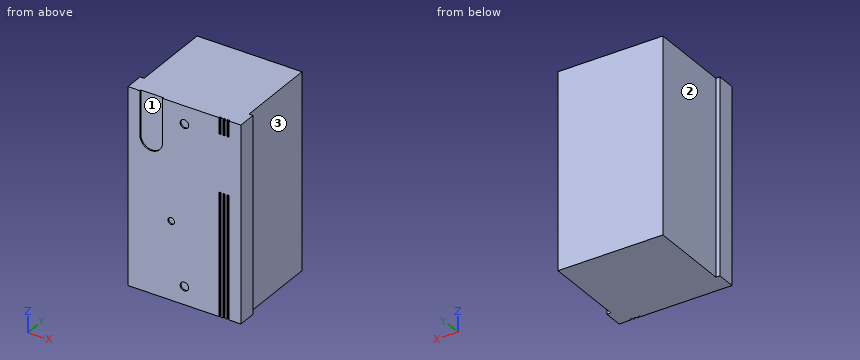
from build123d import *

# Parameters (mm, degrees)
F0_W     = 85
F0_H     = 147
F1_DEPTH = 75
F2_W     = 1.5
F2_H     = 92
F2_R     = 3.213136
F2_R_2   = 2.5
F2_H_2   = 12
F3_DEPTH = 1
F4_W     = 61
F4_H     = 147
F5_DEPTH = 3
F6_W     = 61
F6_H     = 147
F7_DEPTH = 3


with BuildPart() as f1:
    # F0 (on Front) → F1 (new body)
    with BuildSketch(Plane.XZ):
        Rectangle(F0_W, F0_H)
    extrude(amount=F1_DEPTH)

    # F2 (on face) → F3 (cut)
    with BuildSketch(Plane.XZ.offset(75)):
        with Locations((26.781611, -27.5)):
            Rectangle(F2_W, F2_H)
        with Locations((29.781611, -27.5)):
            Rectangle(F2_W, F2_H)
        with Locations((32.781611, -27.5)):
            Rectangle(F2_W, F2_H)
        with Locations((0, -60)):
            Circle(F2_R)
        with Locations((-10, -15)):
            Circle(F2_R_2)
        with Locations((0, 60)):
            Circle(F2_R)
        with BuildLine():
            Line((-16.484489, 73.5), (-33.484489, 73.5))
            Line((-33.484489, 73.5), (-33.484489, 40.5))
            ThreePointArc((-33.484489, 40.5), (-24.984489, 32), (-16.484489, 40.5))
            Line((-16.484489, 40.5), (-16.484489, 73.5))
        make_face()
        with Locations((26.781611, 67.5)):
            Rectangle(F2_W, F2_H_2)
        with Locations((29.781611, 67.5)):
            Rectangle(F2_W, F2_H_2)
        with Locations((32.781611, 67.5)):
            Rectangle(F2_W, F2_H_2)
    extrude(amount=-F3_DEPTH, mode=Mode.SUBTRACT)

    # F4 (on face) → F5 (cut)
    with BuildSketch(Plane(origin=(-42.5, 0, 0), x_dir=(0, -1, 0), z_dir=(-1, 0, 0))):
        with Locations((30.5, 0)):
            Rectangle(F4_W, F4_H)
    extrude(amount=-F5_DEPTH, mode=Mode.SUBTRACT)

    # F6 (on face) → F7 (cut)
    with BuildSketch(Plane.YZ.offset(42.5)):
        with Locations((-30.5, 0)):
            Rectangle(F6_W, F6_H)
    extrude(amount=-F7_DEPTH, mode=Mode.SUBTRACT)


solid = f1.part
Can you work these out from the model? Positions are in its coordinate system, mm. Face numbers are marked on the shaded views. A direction names the side the tool comes from. Give positions to 0.01 mm unless a question says otherwise; leave off trailing zeros. Write each loop counter-clockwise with the first axis right and the second up, starting at its lowest first coordinate (ties: lowest second). Pieces come first, ordered by that corner, then holes. Notation, with made-up numbers: (-35, 20.25) -> (-29, 20.25) arc R24 cw to (-29, 36.25) -> close; hole circle Ø2 at (56.5, 12.25). An arc over 180 degrees is marked (long way). Answer as a JSON object with one key per item and string values. Group by question number.
Item 1: I'm going to push flat-ended pins straight in: P1, Ø2, axis at y = -45.5, z = -56, coming from the +X side; P2, Ø5, axis at x = 0, z = 60, coming from the -Y side; P3, Ø0.8, axis at x = 33, y = -74.5, coming from the -Z side; P4, Ø1.6, axis at x = 33, z = 68.5, coming from the -Y side. Where does each tip first touch, or does it pass through?
Item 2: Please list where these lines run through material, in increasing order: line 1 (Z direction, x = 0, y = -74.25); line 2 (X direction, y = -37.5, z = 37); line 3 (Z direction, x = -10, y = -74.35). Write a range as [from, to].
Item 3: Suppose I cut it at D-D (z = -15). Please give me the cut outline in (x, y), plus the area to 3 significant figures.
Item 4: Suppose I cut it at A-A (z = 49.5). Please give me the cut outline in (x, y), plus the area to 3 significant figures.
Item 5: Suppose I cut it at C-C (z = -60). Please give me the cut outline in (x, y).
Item 6: For the marked faces 1, 2 and 3, which set-ups out of +Z, -Z, +X, -X, +Y, -Y let a thin tool reach every point of the face, with its end or its side?
Item 7: Suppose I cut it at B-B (z = -43.5). Please give me the cut outline in (x, y), plus the area to 3 significant figures.
Findings:
{
 "1": {"P1": "stops at x = 39.5", "P2": "stops at y = -74", "P3": "stops at z = 18.5", "P4": "stops at y = -75"},
 "2": {"line 1": "z = [-73.5, -63.21], [-56.79, 56.79], [63.21, 73.5]", "line 2": "x = [-39.5, 39.5]", "line 3": "z = [-73.5, -17.5], [-12.5, 73.5]"},
 "3": {"outline": "(-42.5, -75) -> (-12.5, -75) -> (-12.5, -74) -> (-7.5, -74) -> (-7.5, -75) -> (26.03, -75) -> (26.03, -74) -> (27.53, -74) -> (27.53, -75) -> (29.03, -75) -> (29.03, -74) -> (30.53, -74) -> (30.53, -75) -> (32.03, -75) -> (32.03, -74) -> (33.53, -74) -> (33.53, -75) -> (42.5, -75) -> (42.5, -61) -> (39.5, -61) -> (39.5, 0) -> (-39.5, 0) -> (-39.5, -61) -> (-42.5, -61) -> close", "area": "6,000 mm²"},
 "4": {"outline": "(-42.5, -75) -> (-33.48, -75) -> (-33.48, -74) -> (-16.48, -74) -> (-16.48, -75) -> (42.5, -75) -> (42.5, -61) -> (39.5, -61) -> (39.5, 0) -> (-39.5, 0) -> (-39.5, -61) -> (-42.5, -61) -> close", "area": "5,990 mm²"},
 "5": {"outline": "(-42.5, -75) -> (-3.21, -75) -> (-3.21, -74) -> (3.21, -74) -> (3.21, -75) -> (26.03, -75) -> (26.03, -74) -> (27.53, -74) -> (27.53, -75) -> (29.03, -75) -> (29.03, -74) -> (30.53, -74) -> (30.53, -75) -> (32.03, -75) -> (32.03, -74) -> (33.53, -74) -> (33.53, -75) -> (42.5, -75) -> (42.5, -61) -> (39.5, -61) -> (39.5, 0) -> (-39.5, 0) -> (-39.5, -61) -> (-42.5, -61) -> close"},
 "6": {"face 1": "+Z, -Y", "face 2": "+Z, -Z, -X, +Y", "face 3": "+Z, -Z, +X, +Y"},
 "7": {"outline": "(-42.5, -75) -> (26.03, -75) -> (26.03, -74) -> (27.53, -74) -> (27.53, -75) -> (29.03, -75) -> (29.03, -74) -> (30.53, -74) -> (30.53, -75) -> (32.03, -75) -> (32.03, -74) -> (33.53, -74) -> (33.53, -75) -> (42.5, -75) -> (42.5, -61) -> (39.5, -61) -> (39.5, 0) -> (-39.5, 0) -> (-39.5, -61) -> (-42.5, -61) -> close", "area": "6,000 mm²"}
}
